from build123d import *

# Parameters (mm, degrees)
SKETCH1_W                  = 76.2
SKETCH1_H                  = 19.05
BOSS_EXTRUDE1_DEPTH        = 1.5875
SKETCH2_R                  = 3.96875
SKETCH2_R_2                = 2.38125
BOSS_EXTRUDE2_DEPTH        = 76.2
SKETCH4_R                  = 1.5875
CUT_EXTRUDE1_DEPTH         = 41.914713601
CHAMFER1_SIZE              = 0.79375
LPATTERN1_COUNT            = 3
LPATTERN1_PITCH            = 25.4
CHAMFER1_OF_LPATTERN1_SIZE = 0.79375
CUT_EXTRUDE2_DEPTH         = 15.24
LPATTERN2_COUNT            = 5
LPATTERN2_PITCH            = 15.24


with BuildPart() as part:
    # Sketch1 → Boss-Extrude1 (new body)
    with BuildSketch(Plane(origin=(0, 0, 0), x_dir=(1, 0, 0), z_dir=(0, 1, 0))):
        Rectangle(SKETCH1_W, SKETCH1_H)
    extrude(amount=BOSS_EXTRUDE1_DEPTH)

    # Sketch2 → Boss-Extrude2 (add)
    with BuildSketch(Plane(origin=(38.1, 0, 0), x_dir=(0, 0, -1), z_dir=(1, 0, 0))):
        with Locations((-9.525, 3.96875)):
            Circle(SKETCH2_R)
        with Locations((-9.525, 3.96875)):
            Circle(SKETCH2_R_2, mode=Mode.SUBTRACT)
    extrude(amount=-BOSS_EXTRUDE2_DEPTH)

    # Sketch4 → Cut-Extrude1 (cut, through all)
    with BuildSketch(Plane(origin=(0, 1.5875, 0), x_dir=(1, 0, 0), z_dir=(0, 1, 0))):
        with Locations(Location((-25.4, 1.5875, 0), (0, 0, 270))):
            Circle(SKETCH4_R)
    cut_extrude1 = extrude(amount=-CUT_EXTRUDE1_DEPTH, mode=Mode.SUBTRACT)

    # Chamfer1
    chamfer1_edges = [part.edges().sort_by_distance(p)[0] for p in [
        (-25.4, 1.5875, -3.175),
    ]]
    chamfer(chamfer1_edges, length=CHAMFER1_SIZE)

    # LPattern1: Cut-Extrude1 ×3
    with Locations(*[(i * LPATTERN1_PITCH, 0, 0) for i in range(1, LPATTERN1_COUNT)]):
        add(cut_extrude1, mode=Mode.SUBTRACT)

    # Chamfer1 of LPattern1
    chamfer1_of_lpattern1_edges = [part.edges().sort_by_distance(p)[0] for p in [
        (0, 1.5875, -3.175),
        (25.4, 1.5875, -3.175),
    ]]
    chamfer(chamfer1_of_lpattern1_edges, length=CHAMFER1_OF_LPATTERN1_SIZE)

    # Sketch5 → Cut-Extrude2 (cut)
    with BuildSketch(Plane(origin=(38.1, 0, 0), x_dir=(0, 0, -1), z_dir=(1, 0, 0))):
        with BuildLine():
            Line((-6.35, 1.5875), (-6.35, 0))
            Line((-6.35, 0), (-9.525, 0))
            ThreePointArc((-9.525, 0), (-11.299878957, 7.518507914), (-6.35, 1.5875))
        make_face()
    cut_extrude2 = extrude(amount=-CUT_EXTRUDE2_DEPTH, mode=Mode.SUBTRACT)

    # LPattern2: Cut-Extrude2 ×5, 2 skipped
    with Locations(*[(-i * LPATTERN2_PITCH, 0, 0) for i in range(1, LPATTERN2_COUNT) if i not in (1, 3)]):
        add(cut_extrude2, mode=Mode.SUBTRACT)


solid = part.part
Source: CAD feature listing. Evaluate the final solid. Frame: model axes, mm. A direction names the side the tool comes from. Round coordinates to 2 decimals unless told otherwise and drop trailing zeros. Loops run counter-clockwise (first coordinate to the right, second up) from the corner with the lowest first, then second, coordinate; pieces in that order, holes last. Notation, with made-up numbers: (-31, -31) - (-1, -31) arc R29 cw to (-1, -3) - close; hole circle Ø10 at (59.25, -26.75). An arc over 180 degrees is marked (long way). Write item = value, one per line. Start each with the question number.
Item 1: Material intervals for line 1 (X direction, y = 1.5, z = 11); line 2 (Y direction, x = 15.5, z = -8.25); line 3 (Z direction, x = -5.5, y = 1) (3 decimals), sorted ascending.
Item 2: Mould query, pull axis X, two halves, no side actions, for faces 5 (the face through (-1, 0, 2)), 6 (the face through (0.477, 0.402, -0.073)), 7 (the face through (38.1, 1, -1)), 8 (the face through (7.62, 1, 9)). Classes: released by +X, released by -X, zero draft, split by the parting line, or undercut.
Item 3: Reachability of faces 1 (the face through (0, 1, 6.35)), 2 (the face through (-30, 1, 6.35)), 3 (the face through (31, 1, 6.35)), 4 (the face through (-24.061, 0.402, -0.734)) from +Z, -Z, +X, -X, +Y, -Y: full face, straight path, thin tool, end or side. Return the list, or none.
Item 4: First-contact query: pin 1 Ø2 at (x, y) = (-19, 2) entering from +Z; pin 2 Ø3 at (y, z) = (1.5, 11) entering from -X; pin 3 Ø4 at (y, z) = (3.97, 9.52) entering from -X; pin 4 Ø4 at (x, z) = (0, -1.59) entering from +Y. Flat tips, straight axial feed; report the tip coordinate or a pass-through.
Item 5: Section query B-B on y = 2.75. Output: boundary loops of the cut face in (x, z), plus the area to 3 significant figures.
Results list:
q1.line_1 = -22.86 to -7.62, 7.62 to 22.86
q1.line_2 = 0 to 1.59
q1.line_3 = -9.525 to 6.35
q2.face_5 = zero draft
q2.face_6 = undercut
q2.face_7 = released by +X
q2.face_8 = undercut
q3.face_1 = +Z, +Y, -Y
q3.face_2 = +Z, -X, +Y, -Y
q3.face_3 = +Z, +X, +Y, -Y
q3.face_4 = +Y, -Y
q4.pin_1 = 13.37
q4.pin_2 = -22.86
q4.pin_3 = through
q4.pin_4 = 1.21
q5.outline = (-22.86, 5.75) - (-7.62, 5.75) - (-7.62, 7.48) - (-22.86, 7.48) - close; (-22.86, 11.57) - (-7.62, 11.57) - (-7.62, 13.3) - (-22.86, 13.3) - close; (7.62, 5.75) - (22.86, 5.75) - (22.86, 7.48) - (7.62, 7.48) - close; (7.62, 11.57) - (22.86, 11.57) - (22.86, 13.3) - (7.62, 13.3) - close
q5.area = 106 mm²
